```python
from build123d import *

# Parameters (mm, degrees)
F1_DEPTH = 68.2625
F2_R     = 7.9375
F2_R_2   = 7.14375
F2_R_3   = 7.1501
F3_DEPTH = 25.4
F4_R     = 3.96875
F5_DEPTH = 25.4


with BuildPart() as f1:
    # F0 (on Front) → F1 (new body, symmetric)
    with BuildSketch(Plane.XZ):
        with BuildLine():
            Line((-19.05, 20.6375), (19.05, 20.6375))
            ThreePointArc((19.05, 20.6375), (20.172532, 20.172532), (20.6375, 19.05))
            Line((20.6375, 19.05), (20.6375, -20.6375))
            Line((20.6375, -20.6375), (20.6375, -26.9875))
            Line((20.6375, -26.9875), (26.9875, -26.9875))
            Line((26.9875, -26.9875), (26.9875, 25.4))
            ThreePointArc((26.9875, 25.4), (26.522532, 26.522532), (25.4, 26.9875))
            Line((25.4, 26.9875), (-25.4, 26.9875))
            ThreePointArc((-25.4, 26.9875), (-26.522532, 26.522532), (-26.9875, 25.4))
            Line((-26.9875, 25.4), (-26.9875, -26.9875))
            Line((-26.9875, -26.9875), (-20.6375, -26.9875))
            Line((-20.6375, -26.9875), (-20.6375, -20.6375))
            Line((-20.6375, -20.6375), (-20.6375, 19.05))
            ThreePointArc((-20.6375, 19.05), (-20.172532, 20.172532), (-19.05, 20.6375))
        make_face()
    extrude(amount=F1_DEPTH, both=True)

    # F2 (on face) → F3 (cut)
    with BuildSketch(Plane.XY.offset(26.9875)):
        Circle(F2_R)
        with Locations((0, 47.625)):
            Circle(F2_R_2)
        with Locations((0, -47.625)):
            Circle(F2_R_3)
    extrude(amount=-F3_DEPTH, mode=Mode.SUBTRACT)

    # F4 (on face) → F5 (cut)
    with BuildSketch(Plane.YZ.offset(26.9875)):
        with Locations((-32.54375, 0)):
            Circle(F4_R)
        with Locations((24.60625, 0)):
            Circle(F4_R)
    extrude(amount=-F5_DEPTH, mode=Mode.SUBTRACT)


solid = f1.part
```
Check sheet for the modelled part. Datum: model origin and axes. Units: mm. A direction names the side the tool comes from. Round coordinates to 2 decimals unless told otherwise and drop trailing zeros. Order: outer loops, then holes, each group sorted by start corner. A loop starts at its lowest first (then second) coordinate and runs counter-clockwise, first axis right, second up. Notation, with made-up numbers: (56.5, 83.5) -> (91.5, 83.5) arc R20 cw to (91.5, 93.5) -> close; hole circle Ø8 at (65, -24.75). An arc over 180 degrees is marked (long way). One line per item, written item: value. Start each with the question number.
Q1. Set-up check for faces 1 (the face through (-2, 68.262, 22)), 2 (the face through (-20.638, -1, -4)), 3 (the face through (23.86, -36.51, 0.17)): record each of +Z, -Z, +X, -X, +Y, -Y from which the full face is reachable in a straight line by a thin tool's end or side.
Q2. Gauge pin test, flat ends, axial feed: pin 1 Ø5 at (y, z) = (-32.54, 0) entering from +X; pin 2 Ø14.5 at (x, y) = (0, 0) entering from -Z; pin 3 Ø19 at (x, y) = (-0.5, -12) entering from -Z. Record the tip position at first contact, or that the pin passes through.
Q3. Cross-section at B-B (x = 0). Record the boundary of the cut face in (y, z).
Q4. Cross-section at D-D (z = 0). Record the boundary of the cut face in (x, y) (1 decimal), and give its area (3 significant figures).
Q5. Mould release check, pull along X, two halves, no side actions. Record for faces 4 (the face through (26.988, -1, -1)), 5 (the face through (-0.931, -40.536, 23.857)), 6 (the face through (23.857, 28.272, -1.52)): pulls with the +X half, pulls with the -X half, needs draft (parallel to the pull), parting line crosses it, or undercut.
Q6. Cross-section at A-A (z = 12). Record the boundary of the cut face in (x, y), and give its area (3 significant figures).
Q7. Thickness scan on line 1 (Y direction, x = 0, z = 24.25); line 2 (X direction, y = 57, z = -7); line 3 (Z direction, x = -15, y = -1). Record the ranges inside material, lowest first.
Completed:
1. face 1: +Z, -Z, +X, -X, +Y
1. face 2: -Z, +Y, -Y
1. face 3: +X
2. pin 1: stops at x = -20.64
2. pin 2: passes through
2. pin 3: stops at z = 20.64
3. outline: (-68.26, 20.64) -> (-54.78, 20.64) -> (-54.78, 26.99) -> (-68.26, 26.99) -> close; (-40.47, 20.64) -> (-7.94, 20.64) -> (-7.94, 26.99) -> (-40.47, 26.99) -> close; (7.94, 20.64) -> (40.48, 20.64) -> (40.48, 26.99) -> (7.94, 26.99) -> close; (54.77, 20.64) -> (68.26, 20.64) -> (68.26, 26.99) -> (54.77, 26.99) -> close
4. outline: (-27, -68.3) -> (-20.6, -68.3) -> (-20.6, 68.3) -> (-27, 68.3) -> close; (20.6, -68.3) -> (27, -68.3) -> (27, -36.5) -> (20.6, -36.5) -> close; (20.6, -28.6) -> (27, -28.6) -> (27, 20.6) -> (20.6, 20.6) -> close; (20.6, 28.6) -> (27, 28.6) -> (27, 68.3) -> (20.6, 68.3) -> close
4. area: 1,630 mm²
5. face 4: pulls with the +X half
5. face 5: undercut
5. face 6: needs draft
6. outline: (-26.99, -68.26) -> (-20.64, -68.26) -> (-20.64, 68.26) -> (-26.99, 68.26) -> close; (20.64, -68.26) -> (26.99, -68.26) -> (26.99, 68.26) -> (20.64, 68.26) -> close
6. area: 1,730 mm²
7. line 1: y = -68.26 to -54.78, -40.47 to -7.94, 7.94 to 40.48, 54.77 to 68.26
7. line 2: x = -26.99 to -20.64, 20.64 to 26.99
7. line 3: z = 20.64 to 26.99
